Design review of the part built by this model. Coordinates are the model's own, in mm. Face numbers are marked on the shaded views. A direction names the side the tool comes from. Give positions to 0.01 mm unless a question says otherwise; leave off trailing zeros. Order: outer loops, then holes, each group sorted by start corner. A loop starts at its lowest first (then second) coordinate and runs counter-clockwise, first axis right, second up. Notation, with made-up numbers: (60, 28.5) -> (94, 28.5) arc R23 ccw to (94, 49.5) -> close; hole circle Ø1 at (1.5, 25.5). An arc over 180 degrees is marked (long way). One line per item, written item: value. Start each with the question number.
1) For pin 1 (2 mm diameter, centred on x = 3, z = 0.5, fed in from -Y); pin 2 (4 mm diameter, centred on x = 3.5, z = -0.5, fed in from +Y); pin 3 (1 mm diameter, centred on x = 4, y = 3, fed in from -Z), all flat-tipped, find the tip position at first contact; note any pin that passes through.
2) Consider section D-D (z = -4.25). State the section outline as (x, y) points.
3) The part is to be moulded in two halves that separate along Z. For the marked faces 3, 4 and 5, say which applies: released by +Z, released by -Z, zero draft, split by the parting line, or undercut.
4) Wall thickness on line 1 along Z through (x, y) = (2.5, 0) (3 decimals); line 2 along X through (y, z) = (-2, -5.5); line 3 along Y through (x, z) = (4.75, 1.5): over which ranges is each line inside the solid? List them lowest first. Write a range as from..to.
5) Consider section C-C (x = 0.5). State the section outline as (y, z) points (3 decimals).
6) Tool access review of the marked faces 1 and 2: name each direction out of +Z, -Z, +X, -X, +Y, -Y from which nothing blocks a thin tool from reaching the whole face with its end or side.
7) Consider section A-A (z = 0). State the section outline as (x, y) points (3 decimals).
Autodesk Inventor part; units mm, degrees
ref_plane "YZ Plane" through (0, 0, 0) normal (1, 0, 0) x (0, 1, 0)
ref_plane "XZ Plane" through (0, 0, 0) normal (0, 1, 0) x (-1, 0, 0)
ref_plane "XY Plane" through (0, 0, 0) normal (0, 0, 1) x (1, 0, 0)
sketch "Sketch_1" plane through (0, 0, 0) normal (0, 0, 1) x (1, 0, 0)
  line L0 (7, 0) -> (0, 0)
  line L1 (0, 3.3) -> (0.3, 3)
  line L2 (0.3, 3) -> (6.7, 3)
  line L3 (6.7, 3) -> (7, 3.3)
  line L4 (7, 3.3) -> (7, 3.7)
  line L5 (7, 3.7) -> (6, 4)
  line L6 (6, 4) -> (1, 4)
  line L7 (1, 4) -> (1, 6)
  line L8 (1, 6) -> (0, 6)
  line L9 (0, 6) -> (0, 3.3)
revolve "Revolution1" add sketch "Sketch_1" angle 360 about axis through (7, 0, 0) along (1, 0, 0)
sketch "스케치2" plane through (0, 0, 0) normal (-1, 0, 0) x (0, 0, 1)
  circle A0 centre (0, 0) radius 3.3
  circle A1 centre (0, 0) radius 6
  circle A2 centre (0, 0) radius 3.025
  dimension "d1" = 6.05
extrude "돌출1" cut sketch "스케치2" against normal up to surface (7 mm away) contours A2
properties part number "80F-0606"
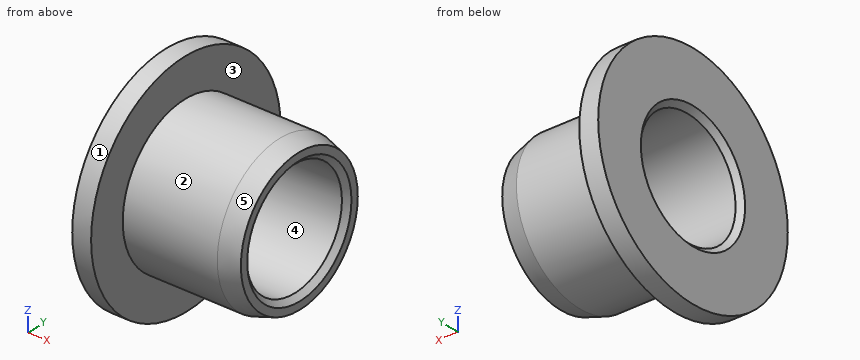
Checked values:
1. pin 1: stops at y = -4
1. pin 2: stops at y = 4
1. pin 3: stops at z = -3.12
2. outline: (0, -4.24) -> (1, -4.24) -> (1, 4.24) -> (0, 4.24) -> close
3. face 3: zero draft
3. face 4: undercut
3. face 5: split by the parting line
4. line 1: z = -4..-3.025, 3.025..4
4. line 2: x = 0..1
4. line 3: y = -3.71..-2.63, 2.63..3.71
5. outline: circle Ø12 at (0, 0); hole circle Ø6.05 at (0, 0)
6. face 1: +X, -X
6. face 2: +X
7. outline: (0, -6) -> (1, -6) -> (1, -4) -> (6, -4) -> (7, -3.7) -> (7, -3.3) -> (6.725, -3.025) -> (0.275, -3.025) -> (0, -3.3) -> close; (0, 3.3) -> (0.275, 3.025) -> (6.725, 3.025) -> (7, 3.3) -> (7, 3.7) -> (6, 4) -> (1, 4) -> (1, 6) -> (0, 6) -> close
